Could you check a few things on this model? Use its own coordinates, in mm. A direction names the side the tool comes from. Coordinates: 2 decimals unless noted, no trailing zeros. Write each loop counter-clockwise with the first axis right and the second up, starting at its lowest first coordinate (ties: lowest second). Pieces come first, ordered by that corner, then holes.
Autodesk Inventor part; units mm, degrees
ref_plane "YZ Plane" through (0, 0, 0) normal (1, 0, 0) x (0, 1, 0)
ref_plane "XZ Plane" through (0, 0, 0) normal (0, 1, 0) x (-1, 0, 0)
ref_plane "XY Plane" through (0, 0, 0) normal (0, 0, 1) x (1, 0, 0)
sketch "Sketch1" plane through (0, 0, 0) normal (0, 1, 0) x (-1, 0, 0)
  line L0 (250, 0) -> (-250, 0)
  line L1 (-250, 0) -> (-250, 380)
  line L2 (-250, 380) -> (250, 380)
  line L3 (250, 380) -> (250, 0)
  point P0 (0, 0)
  point P1 (0, 0)
  dimension "d0" = 500
  dimension "d1" = 380
extrude "Extrusion1" add sketch "Sketch1" along normal blind 280
fillet "Fillet1" radius 20 4 edges at (-250, 280, 190) (-250, 0, 190) (250, 0, 190) (250, 280, 190)
sketch "Sketch2" plane through (-230, 0, 380) normal (0, 0, 1) x (1, 0, 0)
  line L0 (460, 280) -> (0, 280)
  line L1 (360, 280) -> (360, 0)
  line L2 (480, 20) -> (480, 260)
  line L3 (0, 0) -> (460, 0)
  point P0 (230, 0)
  dimension "d5" = 120
split_face "Split1"
sketch "Sketch3" plane through (0, 0, 0) normal (0, -1, 0) x (1, 0, 0)
  circle A0 centre (-190, 340) radius 15
  line L0 (230, 380) -> (230, 0)
  line L1 (130, 380) -> (230, 380)
  line L2 (-230, 380) -> (130, 380)
  line L3 (-230, 0) -> (-230, 380)
  line L4 (230, 0) -> (-230, 0)
  line L5 (130, 340) -> (190, 340) construction
  line L6 (190, 340) -> (190, 40) construction
  line L7 (190, 40) -> (-190, 40) construction
  line L8 (-190, 40) -> (-190, 340) construction
  line L9 (-190, 340) -> (130, 340) construction
  circle A1 centre (-190, 40) radius 15
  circle A2 centre (190, 40) radius 15
  circle A3 centre (190, 340) radius 15
  point P0 (0, 0)
  dimension "d6" = 30
  dimension "d7" = 40
extrude "Extrusion2" add sketch "Sketch3" along normal blind 25 contours A0 | A1 | A2 | A3
properties part number "Microonde" material "Steel, Galvanized"
1. If we mould it in two halves opening along Z, with no side actions, what happens to faces 3 (the face through (-3, 138, 0)), 4 (the face through (-204.985, -12.325, 39.34)), 5 (the face through (190, -25, 340))? For each: pulls with the +Z half, pulls with the -Z half, needs draft (parallel to the pull), parting line crosses it, or undercut.
Verdict:
face 3: pulls with the -Z half
face 4: undercut
face 5: needs draft
2. I want a section at D-D on x = 99. Please give me the cut outline in (y, z), plus the area to 3 significant figures.
Verdict:
outline: (0, 0) - (280, 0) - (280, 380) - (0, 380) - close
area: 106,000 mm2
3. For pin 1 (5 mm diameter, centred on x = -104, z = 295.5, fed in from -Y); pin 2 (8 mm diameter, centred on y = 8.5, z = 184.5, fed in from -X), each with a flat end and sliding along its axis, tell me the tip position at first contact or that it passes through.
Verdict:
pin 1: stops at y = 0
pin 2: stops at x = -248.54
4. I want a section at B-B on z = 40. Please give me the cut outline in (x, y), plus the area to 3 significant figures.
Verdict:
outline: (-250, 20) arc R20 ccw to (-230, 0) - (-205, 0) - (-205, -25) - (-175, -25) - (-175, 0) - (175, 0) - (175, -25) - (205, -25) - (205, 0) - (230, 0) arc R20 ccw to (250, 20) - (250, 260) arc R20 ccw to (230, 280) - (-230, 280) arc R20 ccw to (-250, 260) - close
area: 141,000 mm2
5. On a 3-axis mill with a long thin cutter (end or side, diameter ignored), from which of +Z, -Z, +X, -X, +Y, -Y can I reach the whole of each face in a straight line? I mean faces 1 (the face through (-243.986, 5.703, 187.34)), 2 (the face through (-191.953, -12.325, 325.128)). Say none if no direction works.
Verdict:
face 1: +Z, -Z, -X, -Y
face 2: -Y
6. Please list where these lines run through material, in increasing order: line 1 along Y through (x, z) = (88, 50); line 2 along X through (y, z) = (12, 139).
Verdict:
line 1: y = 0 to 280
line 2: x = -248.33 to 248.33
7. I want a section at C-C on z = 188. Please give me the cut outline in (x, y).
Verdict:
outline: (-250, 20) arc R20 ccw to (-230, 0) - (230, 0) arc R20 ccw to (250, 20) - (250, 260) arc R20 ccw to (230, 280) - (-230, 280) arc R20 ccw to (-250, 260) - close
8. I want a section at A-A on x = 190. Please give me the cut outline in (y, z).
Verdict:
outline: (-25, 25) - (0, 25) - (0, 0) - (280, 0) - (280, 380) - (0, 380) - (0, 355) - (-25, 355) - (-25, 325) - (0, 325) - (0, 55) - (-25, 55) - close
